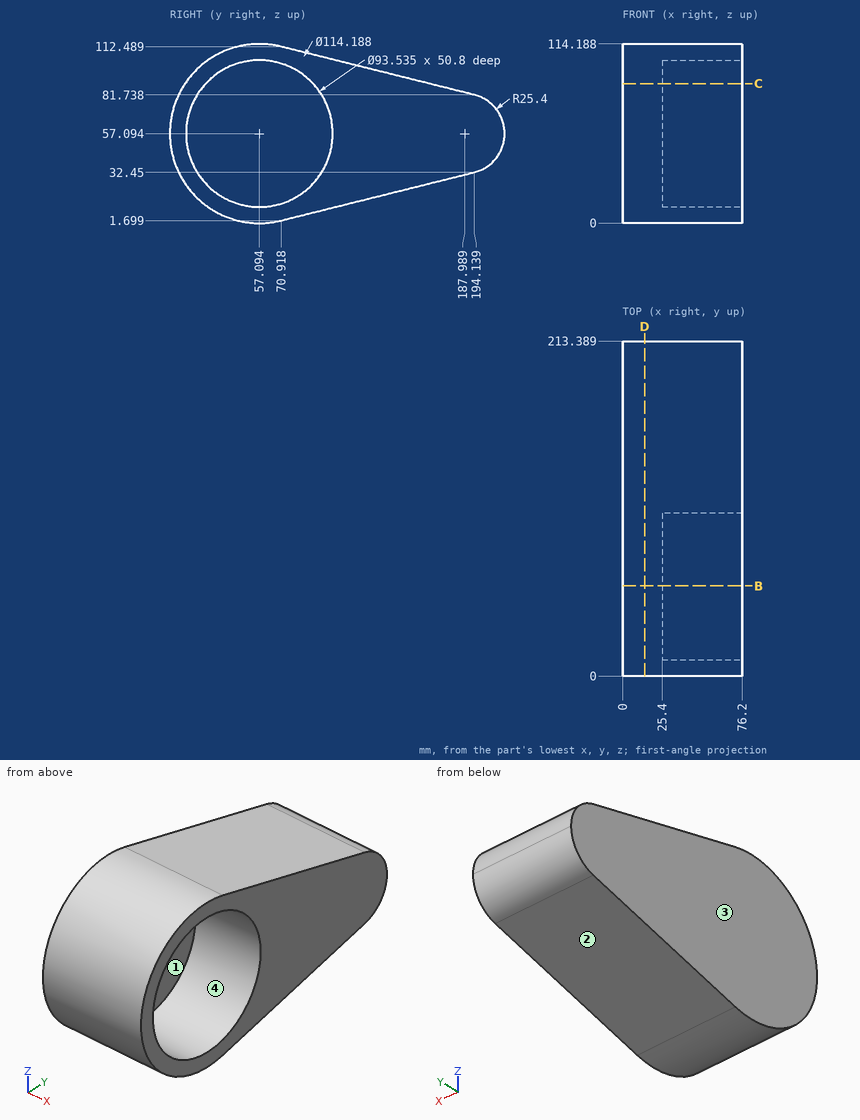
Print and shaded views of the part. All mm, measured from the part's lowest x, y and z. Give positions to 0.01 mm unless a question says otherwise; leave off trailing zeros. Loops run counter-clockwise (first coordinate to the right, second up) from the corner with the lowest first, then second, coordinate; pieces in that order, holes last.
1) Saw through at B-B (y = 57.5). Write the cut outline in (x, z), plus the area to 3 significant figures.
2) Wall check: line 1 (X direction, y = 77, z = 93.5); line 2 (Y direction, x = 31.5, z = 65); line 3 (Y direction, x = 26.5, z = 37) (1 decimal). Give the ranges that are in metal, low to high.
3) Saw through at D-D (x = 14). Write the cut outline in (y, z), plus the area to 4 significant figures.
4) Saw through at C-C (z = 89). Write the cut outline in (x, y).
5) Pull direction Y, two halves, no side cores. Call the marked faces 1, 2, 3 and 4: +Y half, -Y half, draft (parallel to the pull), parting line (faces both ways), or undercut.
6) Flat gauge pins, fed straight in: pin 1 Ø12 at (y, z) = (121.5, 26.5) entering from -X; pin 2 Ø2 at (x, y) = (15.5, 120.5) entering from -Z; pin 3 Ø4 at (x, z) = (44, 51) entering from +Y; pin 4 Ø2 at (x, z) = (39.5, 62.5) entering from +Y. Where does each tip first touch, or does it go through?
Answer block:
1. outline: (0, 0) - (76.2, 0) - (76.2, 10.33) - (25.4, 10.33) - (25.4, 103.86) - (76.2, 103.86) - (76.2, 114.19) - (0, 114.19) - close
1. area: 3,950 mm2
2. line 1: x = 0 to 25.4
2. line 2: y = 0.55 to 11, 103.19 to 212.13
2. line 3: y = 3.7 to 14.9, 99.3 to 203.5
3. outline: (70.92, 1.7) - (194.14, 32.45) arc R25.4 ccw to (194.14, 81.74) - (70.92, 112.49) arc R57.09 ccw (long way) to start
3. area: 17,250 mm2
4. outline: (0, 9.75) - (76.2, 9.75) - (76.2, 22.9) - (25.4, 22.9) - (25.4, 91.29) - (76.2, 91.29) - (76.2, 165.04) - (0, 165.04) - close
5. face 1: undercut
5. face 2: +Y half
5. face 3: draft
5. face 4: undercut
6. pin 1: stops at x = 0
6. pin 2: stops at z = 13.82
6. pin 3: stops at y = 213.06
6. pin 4: stops at y = 213
